Can you work these out from the model? Positions are in its coordinate system, mm. A direction names the side the tool comes from. Coordinates: 2 decimals unless noted, no trailing zeros. Order: outer loops, then holes, each group sorted by start corner. A loop starts at its lowest first (then second) coordinate and runs counter-clockwise, first axis right, second up. Notation, with made-up numbers: (79, -27.75) - (97, -27.75) arc R24 cw to (97, -10.75) - close; hole circle Ø11 at (71.25, -22.5). An arc over 180 degrees is marked (long way). Return JSON: item names as keys, results as strings. Group by question number.
1) For pin 1 Ø4 at (x, y) = (-1.5, -41) entering from +Z (3 decimals); pin 2 Ø3 at (x, z) = (-8, -62.5) entering from -Y; pin 3 Ø22 at (x, z) = (-34.5, -34) entering from +Y (3 decimals); pin 4 Ø9.5 at (y, z) = (31, -30) entering from -X, each with a flat end and sliding along its axis, tell me the tip position at first contact or that it passes through.
2) Imagine slicing it at C-C (z = -4.5). Write out the boundary of the cut face in (x, y) (3 decimals).
3) Imagine slicing it at A-A (z = -12.7). Give the number of separate pieces and of enclosed holes in the cut face, and give its area (3 significant figures).
4) Imagine slicing it at B-B (y = 25.5). Write out the boundary of the cut face in (x, z) (3 decimals), and give its area (3 significant figures).
5) If we mould it in two halves opening along Y, with no side actions, what happens to faces 1 (the face through (1.61, 24.468, -14.632)), 2 (the face through (11, 41.275, 1)), 3 (the face through (-50.8, 2, -34))? For each: pulls with the +Y half, pulls with the -Y half, needs draft (parallel to the pull), parting line crosses it, or undercut.
6) If I drill on line 1 along X through (y, z) = (16.5, -46) (3 decimals), over which ranges is the centre line in solid material (lowest first)?
7) Imagine slicing it at D-D (x = -28). Write out the boundary of the cut face in (y, z) (3 decimals), and give its area (3 significant figures).
8) Which directions (+Z, -Z, +X, -X, +Y, -Y) give clear straight access to the entire face, cutting with the end or side of a thin tool? Please do faces 4 (the face through (3.175, -28, -35)), 5 (the face through (0, 22, -27)), 6 (the face through (2, -50.8, -34)), 7 (the face through (18, 3.175, -28)).
```python
from build123d import *

# Parameters (mm, degrees)
F0_W          = 50.8
F0_H          = 50.8
F1_DEPTH      = 3.175
F2_W          = 50.8
F2_H          = 3.175
F3_DEPTH      = 12.7
F3_DEPTH_BACK = 76.2
F4_W          = 3.175
F4_H          = 101.6
F5_DEPTH      = 12.7
F5_DEPTH_BACK = 76.2
F7_W          = 47.625
F7_H          = 12.7
F8_DEPTH      = 25.4
F9_W          = 47.625
F9_H          = 12.7
F10_DEPTH     = 25.4
F12_DEPTH     = 25.4
F14_DEPTH     = 25.4
F16_DEPTH     = 53.976
F18_DEPTH     = 76.2
F19_R         = 3.175
F20_DEPTH     = 25.4
F21_R         = 3.175
F22_DEPTH     = 25.4
F23_R         = 3.175
F24_DEPTH     = 25.4
F26_DEPTH     = 76.201


with BuildPart() as f1:
    # F0 (on Top) → F1 (new body)
    with BuildSketch(Plane.XY):
        with Locations((25.4, 25.4)):
            Rectangle(F0_W, F0_H)
    extrude(amount=F1_DEPTH)

    # F2 (on face) → F3 (join, two sides)
    with BuildSketch(Plane.XY.offset(3.175)) as f3_sk:
        with Locations((-25.4, 1.5875)):
            Rectangle(F2_W, F2_H)
        with Locations((25.4, 1.5875)):
            Rectangle(F2_W, F2_H)
    extrude(amount=F3_DEPTH)
    extrude(f3_sk.sketch, amount=-F3_DEPTH_BACK)

    # F4 (on face) → F5 (join, two sides)
    with BuildSketch(Plane.XY.offset(3.175)) as f5_sk:
        with Locations((1.5875, 0)):
            Rectangle(F4_W, F4_H)
    extrude(amount=F5_DEPTH)
    extrude(f5_sk.sketch, amount=-F5_DEPTH_BACK)

    # F7 (on face) → F8 (cut)
    with BuildSketch(Plane.YZ.offset(3.175)):
        with Locations((26.9875, 9.525)):
            Rectangle(F7_W, F7_H)
    extrude(amount=-F8_DEPTH, mode=Mode.SUBTRACT)

    # F9 (on face) → F10 (cut)
    with BuildSketch(Plane(origin=(0, 3.175, 0), x_dir=(-1, 0, 0), z_dir=(0, 1, 0))):
        with Locations((-26.9875, 9.525)):
            Rectangle(F9_W, F9_H)
    extrude(amount=-F10_DEPTH, mode=Mode.SUBTRACT)

    # F11 (on face) → F12 (cut)
    with BuildSketch(Plane.XZ):
        Polygon((50.8, -6.35), (15.875, -73.025), (50.8, -73.025), align=None)
    extrude(amount=-F12_DEPTH, mode=Mode.SUBTRACT)

    # F13 (on face) → F14 (cut)
    with BuildSketch(Plane(origin=(0, 0, 0), x_dir=(0, -1, 0), z_dir=(-1, 0, 0))):
        Polygon((-15.875, -73.025), (-50.8, -6.35), (-50.8, -73.025), align=None)
    extrude(amount=-F14_DEPTH, mode=Mode.SUBTRACT)

    # F15 (on face) → F16 (cut, through all)
    with BuildSketch(Plane(origin=(0, 3.175, 0), x_dir=(-1, 0, 0), z_dir=(0, 1, 0))):
        Polygon((50.8, 15.875), (-3.175, 15.875), (-3.175, 3.175), (0, 3.175), (50.8, 3.175), align=None)
    extrude(amount=-F16_DEPTH, mode=Mode.SUBTRACT)

    # F17 (on face) → F18 (join, through all)
    with BuildSketch(Plane.XY.offset(3.175)):
        Polygon((9.525, 0), (3.175, 0), (3.175, -6.35), align=None)
        Polygon((-6.35, 3.175), (0, 3.175), (0, 9.525), align=None)
    extrude(amount=-F18_DEPTH)

    # F19 (on face) → F20 (cut)
    with BuildSketch(Plane(origin=(0, 3.175, 0), x_dir=(-1, 0, 0), z_dir=(0, 1, 0))):
        with Locations((-26.9875, -12.7)):
            Circle(F19_R)
    extrude(amount=-F20_DEPTH, mode=Mode.SUBTRACT)

    # F21 (on face) → F22 (cut)
    with BuildSketch(Plane.YZ.offset(3.175)):
        with Locations((26.9875, -12.7)):
            Circle(F21_R)
    extrude(amount=-F22_DEPTH, mode=Mode.SUBTRACT)

    # F23 (on face) → F24 (cut)
    with BuildSketch(Plane(origin=(0, 0, 0), x_dir=(1, 0, 0), z_dir=(0, 0, -1))):
        with Locations((26.9875, -26.9875)):
            Circle(F23_R)
    extrude(amount=-F24_DEPTH, mode=Mode.SUBTRACT)

    # F25 (on face) → F26 (cut, through all)
    with BuildSketch(Plane.XY.offset(3.175)):
        Polygon((41.275, 0), (50.8, 0), (50.8, 50.8), (41.275, 50.8), (0, 50.8), (0, 41.275), (41.275, 41.275), align=None)
    extrude(amount=-F26_DEPTH, mode=Mode.SUBTRACT)


solid = f1.part
```
Calculated:
{
 "1": {"pin 1": "z = 3.175", "pin 2": "y = 0", "pin 3": "y = 3.175", "pin 4": "x = 0"},
 "2": {"outline": "(-50.8, 0) - (0, 0) - (0, -50.8) - (3.175, -50.8) - (3.175, -6.35) - (9.525, 0) - (41.275, 0) - (41.275, 3.175) - (3.175, 3.175) - (3.175, 41.275) - (0, 41.275) - (0, 9.525) - (-6.35, 3.175) - (-50.8, 3.175) - close"},
 "3": {"separate pieces": "3", "enclosed holes": "0", "area": "575 mm2"},
 "4": {"outline": "(0, -54.65) - (3.175, -54.65) - (3.175, -15.505) - (0, -15.505) - close; (0, -9.895) - (3.175, -9.895) - (3.175, 0) - (24.183, 0) - (24.183, 3.175) - (0, 3.175) - close; (29.792, 0) - (41.275, 0) - (41.275, 3.175) - (29.792, 3.175) - close", "area": "269 mm2"},
 "5": {"face 1": "undercut", "face 2": "pulls with the +Y half", "face 3": "needs draft"},
 "6": {"line 1": "0 to 3.175"},
 "7": {"outline": "(0, -73.025) - (3.175, -73.025) - (3.175, 3.175) - (0, 3.175) - close", "area": "242 mm2"},
 "8": {"face 4": "+Z, -Z, +X, -Y", "face 5": "+Z, -Z, -X, +Y", "face 6": "+Z, -Z, +X, -X, -Y", "face 7": "-Z, +X, +Y"}
}
